For this review, take the finished solid that the model builds, in its own axes (mm). A direction names the side the tool comes from. Coordinates: 2 decimals unless noted, no trailing zeros. Loops run counter-clockwise (first coordinate to the right, second up) from the corner with the lowest first, then second, coordinate; pieces in that order, holes last. Notation, with made-up numbers: (62.25, -6) -> (117.25, -6) arc R29 ccw to (117.25, 19) -> close; hole circle Ø2 at (71, 12). An arc over 180 degrees is marked (long way). Answer in a Markdown table with one row per item.
from build123d import *

# Parameters (mm, degrees)
SKETCH1_R           = 1.27
BOSS_EXTRUDE1_DEPTH = 6.35
SKETCH2_R           = 1.397
BOSS_EXTRUDE2_DEPTH = 0.254


with BuildPart() as part:
    # Sketch1 → Boss-Extrude1 (new body, symmetric)
    with BuildSketch(Plane(origin=(0, 0, 0), x_dir=(1, 0, 0), z_dir=(0, 1, 0))):
        Circle(SKETCH1_R)
    extrude(amount=BOSS_EXTRUDE1_DEPTH, both=True)

    # Sketch2 → Boss-Extrude2 (add)
    with BuildSketch(Plane.XZ.offset(6.35)):
        Circle(SKETCH2_R)
    boss_extrude2 = extrude(amount=BOSS_EXTRUDE2_DEPTH)

    # Mirror1: Boss-Extrude2 across plane
    add(boss_extrude2.mirror(Plane.ZX))


solid = part.part
Item 1: Take a section at C-C, the plane y = 1. State the section outline as (x, z) points, and give its area (3 significant figures).
Worked answers:
| item | result |
|---|---|
| outline | circle Ø2.54 at (0, 0) |
| area | 5.07 mm² |
Item 2: For faces 1 (the cylindrical face through (-0.17, 0.09, -1.26)), 2 (the flat face through (0, -6.604, 0)), list the 3-axis set-ups (+Z, -Z, +X, -X, +Y, -Y) from which the entire face can be reached by the end or side of a thin tool; tool diameter is ignored.
Worked answers:
| item | result |
|---|---|
| face 1 | none |
| face 2 | +Z, -Z, +X, -X, -Y |
Item 3: Take a section at B-B, the plane z = 0. State the section outline as (x, y) points, and give its area (3 significant figures).
Worked answers:
| item | result |
|---|---|
| outline | (-1.4, -6.6) -> (1.4, -6.6) -> (1.4, -6.35) -> (1.27, -6.35) -> (1.27, 6.35) -> (1.4, 6.35) -> (1.4, 6.6) -> (-1.4, 6.6) -> (-1.4, 6.35) -> (-1.27, 6.35) -> (-1.27, -6.35) -> (-1.4, -6.35) -> close |
| area | 33.7 mm² |
Item 4: Take a section at A-A, the plane x = 0. State the section outline as (y, z) points, and give its area (3 significant figures).
Worked answers:
| item | result |
|---|---|
| outline | (-6.6, -1.4) -> (-6.35, -1.4) -> (-6.35, -1.27) -> (6.35, -1.27) -> (6.35, -1.4) -> (6.6, -1.4) -> (6.6, 1.4) -> (6.35, 1.4) -> (6.35, 1.27) -> (-6.35, 1.27) -> (-6.35, 1.4) -> (-6.6, 1.4) -> close |
| area | 33.7 mm² |
Item 5: For L1, parallel to Z at x = 0.15, y = 1.25; L2, parallel to X at y = 5.5, z = 0.6; L3, parallel to X at y = 5.75, z = -0.3, list the stretches that pass through material, from the lowest coordinate up.
Worked answers:
| item | result |
|---|---|
| L1 | -1.26 to 1.26 |
| L2 | -1.12 to 1.12 |
| L3 | -1.23 to 1.23 |
Item 6: Insertion check: pin 1 (1.5 mm diameter, centred on y = 3, z = -1, fed in from -X); pin 2 (1.5 mm diameter, centred on x = 1, y = -1, fed in from -Z); pin 3 (1 mm diameter, centred on x = -0.5, y = 0.5, fed in from -Z). Each pin has a flat end and moves straight along its axis. Give the tip position at first contact, or say it passes through.
Worked answers:
| item | result |
|---|---|
| pin 1 | x = -1.25 |
| pin 2 | z = -1.25 |
| pin 3 | z = -1.27 |
